Can you work these out from the drawing? Everything is in mm from the part's minimum corner. A direction names the side the tool comes from. Give positions to 0.01 mm unless a question says otherwise; leave off trailing zeros. Write each loop counter-clockwise with the first axis right and the second up, starting at its lowest first coordinate (ties: lowest second). Pieces come first, ordered by that corner, then holes. Notation, with made-up numbers: (83.25, -30.75) - (132.25, -30.75) arc R20 cw to (132.25, -23.75) - close; hole circle Ø2 at (-29.5, 13.25). An arc over 180 degrees is marked (long way). Write each question's results on one line, items separated by ' | '. Start each with the question number.
Item 1: Suppose I cut it at D-D on x = 6. List the corners of the cut face in (y, z) for me, then the cut area to 3 significant figures.
Item 2: Suppose I cut it at A-A on y = 55. List the corners of the cut face in (x, z) for me.
Item 3: Please list where these lines run through material, in increasing order: line 1 along Y through (x, z) = (5.75, 2.95); line 2 along Y through (x, z) = (26.5, 0.3); line 3 along Y through (x, z) = (18, 4.3).
Item 4: Suppose I cut it at C-C on z = 4.1. List the corners of the cut face in (x, y) for me.
Item 5: We'd pull the mould along X, two halves only. Please class the marked faces 4, 5, 6 and 7: +X half, -X half, draft (parallel to the pull), parting line (faces both ways), or undercut.
Item 6: Will these pins go through, and if not, where does the flat tip stop? P1, Ø1.5, axis at x = 27.25, y = 17, coming from the +Z side; P2, Ø4, axis at x = 18, y = 32, coming from the -Z side.
Item 7: Which directions (+Z, -Z, +X, -X, +Y, -Y) give clear straight access to the entire face, cutting with the end or side of a thin tool? Please do the marked faces 1, 2 and 3.
Item 8: Suppose I cut it at B-B on x = 27.25. List the corners of the cut face in (y, z) for me.
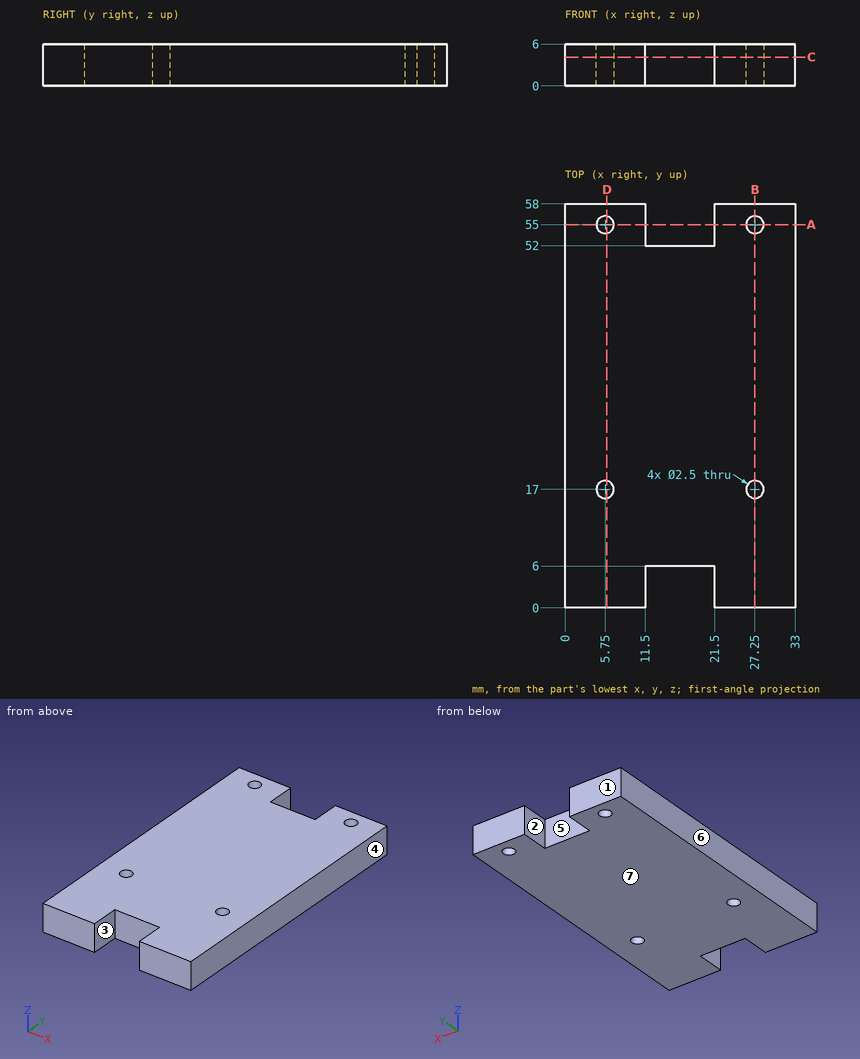
Checked values:
1) outline: (0, 0) - (15.78, 0) - (15.78, 6) - (0, 6) - close; (18.22, 0) - (53.78, 0) - (53.78, 6) - (18.22, 6) - close; (56.22, 0) - (58, 0) - (58, 6) - (56.22, 6) - close | area: 319 mm^2
2) outline: (0, 0) - (4.5, 0) - (4.5, 6) - (0, 6) - close; (7, 0) - (11.5, 0) - (11.5, 6) - (7, 6) - close; (21.5, 0) - (26, 0) - (26, 6) - (21.5, 6) - close; (28.5, 0) - (33, 0) - (33, 6) - (28.5, 6) - close
3) line 1: y = 0 to 15.75, 18.25 to 53.75, 56.25 to 58 | line 2: y = 0 to 16, 18 to 54, 56 to 58 | line 3: y = 6 to 52
4) outline: (0, 0) - (11.5, 0) - (11.5, 6) - (21.5, 6) - (21.5, 0) - (33, 0) - (33, 58) - (21.5, 58) - (21.5, 52) - (11.5, 52) - (11.5, 58) - (0, 58) - close; hole circle Ø2.5 at (5.75, 17); hole circle Ø2.5 at (5.75, 55); hole circle Ø2.5 at (27.25, 17); hole circle Ø2.5 at (27.25, 55)
5) face 4: +X half | face 5: undercut | face 6: -X half | face 7: draft
6) P1: passes through | P2: stops at z = 0
7) face 1: +Z, -Z, +X, -X, +Y | face 2: +Z, -Z, +Y | face 3: +Z, -Z, -Y
8) outline: (0, 0) - (15.75, 0) - (15.75, 6) - (0, 6) - close; (18.25, 0) - (53.75, 0) - (53.75, 6) - (18.25, 6) - close; (56.25, 0) - (58, 0) - (58, 6) - (56.25, 6) - close
